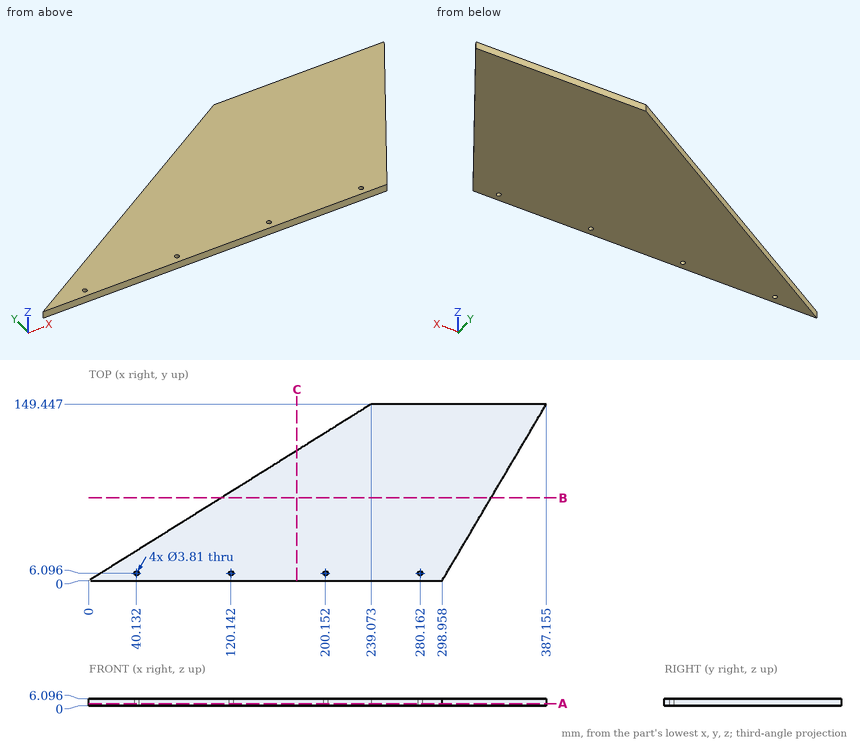
Verification items for this drawing (mm, ordinates from the low corner). Round coordinates to 2 decimals unless told otherwise and drop trailing zeros. Write each loop counter-clockwise with the first axis right and the second up, starting at its lowest first coordinate (ties: lowest second). Pieces come first, ordered by that corner, then holes. Notation, with made-up numbers: M 22,34.5 L 71,34.5 A26 ccw 71,63.5 Z; hole C 49,-2 d8. An arc over 180 degrees is marked long. Write item = value, one per line. Start each with the question number.
1. Gauge pin test, flat ends, axial feed: pin 1 (5 mm diameter, centred on x = 280.162, y = 6.096, fed in from +Z); pin 2 (3 mm diameter, centred on x = 40.132, y = 6.096, fed in from -Z); pin 3 (2 mm diameter, centred on y = 24.5, z = 3, fed in from +X); pin 4 (1 mm diameter, centred on y = 128.5, z = 3, fed in from +X). Record the tip position at first contact, or that the pin passes through.
2. Scan lines: line 1 (Y direction, x = 225, z = 4); line 2 (Y direction, x = 211, z = 4.25); line 3 (X direction, y = 106, z = 1.5) (1 decimal). Record each from-to range of solid material in increasing order. Write a range as [from, to].
3. Section check C-C, the plane x = 176. Record the cut outline in (y, z).
4. Section check A-A, the plane z = 1.75. Record the cut outline in (x, y) (1 decimal), then the cut area to 3 significant figures.
5. Section check B-B, the plane y = 70. Record the cut outline in (x, z).
Results found:
q1.pin_1 = 6.1
q1.pin_2 = through
q1.pin_3 = 314.01
q1.pin_4 = 375.09
q2.line_1 = [0, 140.65]
q2.line_2 = [0, 131.9]
q2.line_3 = [169.6, 361.5]
q3.outline = M 0,0 L 110.02,0 L 110.02,6.1 L 0,6.1 Z
q4.outline = M 0,0 L 299,0 L 387.2,149.4 L 239.1,149.4 Z; hole C 40.1,6.1 d3.8; hole C 120.1,6.1 d3.8; hole C 200.2,6.1 d3.8; hole C 280.2,6.1 d3.8
q4.area = 33,400 mm^2
q5.outline = M 111.98,0 L 340.27,0 L 340.27,6.1 L 111.98,6.1 Z
